Input: part model. Units: mm. Frame: model coordinates. Coordinates: 2 decimals unless noted, no trailing zeros. One line per question, with ' | ' between items.
Autodesk Inventor part; units mm, degrees
ref_plane "C1_XY" through (0, 0, 0) normal (0, 0, 1) x (1, 0, 0)
ref_plane "C1_YZ" through (0, 0, 0) normal (1, 0, 0) x (0, 1, 0)
ref_plane "C1_ZX" through (0, 0, 0) normal (0, 1, 0) x (0, 0, 1)
sketch "Sketch_63" plane through (0, 0, 0) normal (0, 0, 1) x (1, 0, 0)
  line L0 (-10, -7) -> (-8, -7)
  line L1 (-8, -7) -> (-8, -4)
  line L2 (-8, -4) -> (-7.0607, -4)
  line L3 (-7.0607, -4) -> (-4, -7.0607)
  line L4 (-4, -7.0607) -> (-4, -9.4804)
  line L5 (-4, -9.4804) -> (-3.7, -10)
  line L6 (-3.7, -10) -> (-4, -10.5196)
  line L7 (-4, -10.5196) -> (-4, -12.9393)
  line L8 (-4, -12.9393) -> (-7.0607, -16)
  line L9 (-7.0607, -16) -> (-8, -16)
  line L10 (-8, -16) -> (-8, -13)
  line L11 (-8, -13) -> (-10, -13)
  line L12 (-10, -13) -> (-10, -19)
  arc A0 (-10, -19) -> (-9, -20) centre (-9, -19) ccw
  line L13 (-9, -20) -> (-3, -20)
  line L14 (-3, -20) -> (-3, -18)
  line L15 (-3, -18) -> (-6, -18)
  line L16 (-6, -18) -> (-6, -17.0607)
  line L17 (-6, -17.0607) -> (-2.9393, -14)
  line L18 (-2.9393, -14) -> (-0.5196, -14)
  line L19 (-0.5196, -14) -> (0, -13.7)
  line L20 (0, -13.7) -> (0.5196, -14)
  line L21 (0.5196, -14) -> (2.9393, -14)
  line L22 (2.9393, -14) -> (6, -17.0607)
  line L23 (6, -17.0607) -> (6, -18)
  line L24 (6, -18) -> (3, -18)
  line L25 (3, -18) -> (3, -20)
  line L26 (3, -20) -> (9, -20)
  arc A1 (9, -20) -> (10, -19) centre (9, -19) ccw
  line L27 (10, -19) -> (10, 19)
  arc A2 (10, 19) -> (9, 20) centre (9, 19) ccw
  line L28 (9, 20) -> (3, 20)
  line L29 (3, 20) -> (3, 18)
  line L30 (3, 18) -> (6, 18)
  line L31 (6, 18) -> (6, 17.0607)
  line L32 (6, 17.0607) -> (2.9393, 14)
  line L33 (2.9393, 14) -> (0.5196, 14)
  line L34 (0.5196, 14) -> (0, 13.7)
  line L35 (0, 13.7) -> (-0.5196, 14)
  line L36 (-0.5196, 14) -> (-2.9393, 14)
  line L37 (-2.9393, 14) -> (-6, 17.0607)
  line L38 (-6, 17.0607) -> (-6, 18)
  line L39 (-6, 18) -> (-3, 18)
  line L40 (-3, 18) -> (-3, 20)
  line L41 (-3, 20) -> (-9, 20)
  arc A3 (-9, 20) -> (-10, 19) centre (-9, 19) ccw
  line L42 (-10, 19) -> (-10, 13)
  line L43 (-10, 13) -> (-8, 13)
  line L44 (-8, 13) -> (-8, 16)
  line L45 (-8, 16) -> (-7.0607, 16)
  line L46 (-7.0607, 16) -> (-4, 12.9393)
  line L47 (-4, 12.9393) -> (-4, 10.5196)
  line L48 (-4, 10.5196) -> (-3.7, 10)
  line L49 (-3.7, 10) -> (-4, 9.4804)
  line L50 (-4, 9.4804) -> (-4, 7.0607)
  line L51 (-4, 7.0607) -> (-7.0607, 4)
  line L52 (-7.0607, 4) -> (-8, 4)
  line L53 (-8, 4) -> (-8, 7)
  line L54 (-8, 7) -> (-10, 7)
  line L55 (-10, 7) -> (-10, -7)
  line L56 (4, 12.9393) -> (4, 8.5)
  arc A4 (4, 8.5) -> (5, 7.5) centre (5, 8.5) ccw
  line L57 (5, 7.5) -> (7, 7.5)
  arc A5 (7, 7.5) -> (8, 8.5) centre (7, 8.5) ccw
  line L58 (8, 8.5) -> (8, 16)
  line L59 (8, 16) -> (7.0607, 16)
  line L60 (7.0607, 16) -> (4, 12.9393)
  line L61 (4, -12.9393) -> (7.0607, -16)
  line L62 (7.0607, -16) -> (8, -16)
  line L63 (8, -16) -> (8, -8.5)
  arc A6 (8, -8.5) -> (7, -7.5) centre (7, -8.5) ccw
  line L64 (7, -7.5) -> (5, -7.5)
  arc A7 (5, -7.5) -> (4, -8.5) centre (5, -8.5) ccw
  line L65 (4, -8.5) -> (4, -12.9393)
  line L66 (-8, 1.7) -> (-8, -1.7)
  arc A8 (-8, -1.7) -> (-7.7, -2) centre (-7.7, -1.7) ccw
  line L67 (-7.7, -2) -> (-7.0636, -2)
  arc A9 (-6.8515, -2.0879) -> (-7.0636, -2) centre (-7.0636, -2.3) ccw
  line L68 (-6.8515, -2.0879) -> (-2.9393, -6)
  line L69 (-2.9393, -6) -> (7, -6)
  arc A10 (7, -6) -> (8, -5) centre (7, -5) ccw
  line L70 (8, -5) -> (8, 5)
  arc A11 (8, 5) -> (7, 6) centre (7, 5) ccw
  line L71 (7, 6) -> (-2.9393, 6)
  line L72 (-2.9393, 6) -> (-6.8515, 2.0879)
  arc A12 (-7.0636, 2) -> (-6.8515, 2.0879) centre (-7.0636, 2.3) ccw
  line L73 (-7.0636, 2) -> (-7.7, 2)
  arc A13 (-7.7, 2) -> (-8, 1.7) centre (-7.7, 1.7) ccw
extrude "Extrusion1" add sketch "Sketch_63" against normal blind 425
sketch "Sketch2" plane through (0, 0, -425) normal (0, 0, -1) x (-1, 0, 0)
  point P0 (0, 10)
hole "Hole1" at (0, 10, -425) direction (0, 0, 1) diameter 4.2 end through all
pattern_linear "Rectangular Pattern1" count 2 spacing 20 along (0, -1, 0) of "Hole1"
ref_plane "C1_XY" through (0, 0, 0) normal (0, 0, 1) x (1, 0, 0)
ref_plane "C1_YZ" through (0, 0, 0) normal (1, 0, 0) x (0, 1, 0)
ref_plane "C1_ZX" through (0, 0, 0) normal (0, 1, 0) x (0, 0, 1)
thread "Thread1"
thread "Thread2"
thread "Thread3"
thread "Thread4"
properties part number "HFSF5-2040-425" material "Aluminum 6061"
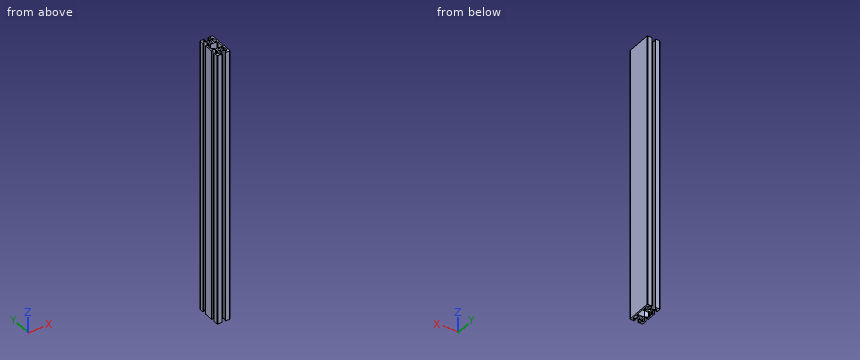
Item 1: Contact query for flat-ended pins moving along their axis: P1, Ø0.7, axis at y = 8, z = -274.5, coming from the -X side; P2, Ø1.5, axis at x = 0, z = -179.5, coming from the +Y side. Output: stop coordinate, or through.
Data:
P1: x = -4 | P2: y = 14
Item 2: Section A-A on z = -175.5. Count the separate pieces of the cut face and the enclosed holes in it, and give its area (3 significant figures).
Data:
separate pieces: 1 | enclosed holes: 5 | area: 343 mm^2
Item 3: Ray query, line 1 (Y direction, x = 0, z = -163); line 2 (X direction, y = 10, z = -172); line 3 (Y direction, x = -7, z = -149.5). Return the intervals inside material, ascending.
Data:
line 1: -13.7 to -12.1, -7.9 to -6, 6 to 7.9, 12.1 to 13.7 | line 2: -3.7 to -2.1, 2.1 to 4, 8 to 10 | line 3: -20 to -15.94, -4.06 to -2.01, 2.01 to 4.06, 15.94 to 20
